```python
from build123d import *

# Parameters (mm, degrees)
SKETCH4_W                          = 6
SKETCH4_H                          = 4.5
BODY_EXTRUDE2_DEPTH                = 6
BODY_SHELL1_T                      = -0.58
BODY_SHELL1_THICKNESS_2_FACE_W     = 3.34
BODY_SHELL1_THICKNESS_2_FACE_H     = 4.84
BODY_SHELL1_THICKNESS_2_DEPTH      = 1.42
EXTRUDE3_REACH                     = 9.075
SKETCH66_W                         = 0.89
SKETCH66_H                         = 1.96
EXTRUDE3_DIRECTION_2_REACH         = 9.075
EXTRUDE2_REACH                     = 9.77
SKETCH65_W                         = 0.5
SKETCH65_H                         = 4
SKETCH65_W_2                       = 1
SKETCH65_H_2                       = 2.5
SKETCH64_W                         = 0.508
SKETCH64_H                         = 0.508
PINS_EXTRUDE_DEPTH                 = 7.045
PINS_CHAMFER_SIZE                  = 0.15
PINS_LPATTERN_COUNT                = 2
PINS_LPATTERN_PITCH                = 2
PINS_CHAMFER_OF_PINS_LPATTERN_SIZE = 0.15


with BuildPart() as part:
    # Sketch4 → Body-Extrude2 (new body)
    with BuildSketch(Plane(origin=(6.86422654, 0, 1.863703399), x_dir=(1, 0, 0), z_dir=(0, 1, 0))):
        with Locations((-6.86422654, 1.863703399)):
            Rectangle(SKETCH4_W, SKETCH4_H)
    extrude(amount=BODY_EXTRUDE2_DEPTH)

    # Body-Shell1
    body_shell1_openings = [part.faces().sort_by_distance(p)[0] for p in [
        (0, 6, 0),
    ]]
    offset(amount=BODY_SHELL1_T, openings=body_shell1_openings, kind=Kind.INTERSECTION)

    # Body-Shell1 thickness 2 face (on inner face of the shell) → Body-Shell1 thickness 2 (add)
    with BuildSketch(Plane(origin=(0, 0.58, 0), x_dir=(0, 0, -1), z_dir=(0, -1, 0))):
        Rectangle(BODY_SHELL1_THICKNESS_2_FACE_W, BODY_SHELL1_THICKNESS_2_FACE_H)
    extrude(amount=-BODY_SHELL1_THICKNESS_2_DEPTH)

    # Extrude3: up to this face of the body (flat: up to its plane)
    extrude3_end = Plane(part.part.faces().sort_by_distance((-3, 3, 0))[0])
    # Sketch66 → Extrude3 (cut, up to the picked face)
    with BuildSketch(Plane(origin=(0, 0, 0), x_dir=(0, 0, -1), z_dir=(1, 0, 0)), mode=Mode.PRIVATE) as extrude3_sk1:
        with Locations((-0.355, 5.02)):
            Rectangle(SKETCH66_W, SKETCH66_H)
    extrude3_tool1 = split(extrude(extrude3_sk1.sketch, amount=-EXTRUDE3_REACH, mode=Mode.PRIVATE), bisect_by=extrude3_end, keep=Keep.BOTH, mode=Mode.PRIVATE)
    add(extrude3_tool1.solids().sort_by(Axis((0, 5.02, 0.355), (-1, 0, 0)))[0], mode=Mode.SUBTRACT)

    # Extrude3 direction 2: up to this face of the body (flat: up to its plane)
    extrude3_direction_2_end = Plane(part.part.faces().sort_by_distance((3, 3, 0))[0])
    # Sketch66 → Extrude3 direction 2 (cut, up to the picked face)
    with BuildSketch(Plane(origin=(0, 0, 0), x_dir=(0, 0, -1), z_dir=(1, 0, 0)), mode=Mode.PRIVATE) as extrude3_direction_2_sk1:
        with Locations((-0.355, 5.02)):
            Rectangle(SKETCH66_W, SKETCH66_H)
    extrude3_direction_2_tool1 = split(extrude(extrude3_direction_2_sk1.sketch, amount=EXTRUDE3_DIRECTION_2_REACH, mode=Mode.PRIVATE), bisect_by=extrude3_direction_2_end, keep=Keep.BOTH, mode=Mode.PRIVATE)
    add(extrude3_direction_2_tool1.solids().sort_by(Axis((0, 5.02, 0.355), (1, 0, 0)))[0], mode=Mode.SUBTRACT)

    # Sketch65 → Extrude2 (cut, up to next)
    with BuildSketch(Plane(origin=(0, 0, 1.67), x_dir=(1, 0, 0), z_dir=(0, 0, -1)), mode=Mode.PRIVATE) as extrude2_sk1:
        with Locations((0, -4)):
            Rectangle(SKETCH65_W, SKETCH65_H)
    extrude2_tool1 = extrude(extrude2_sk1.sketch, amount=-EXTRUDE2_REACH, mode=Mode.PRIVATE) & part.part
    # Sketch65 → Extrude2 (cut, up to next)
    with BuildSketch(Plane(origin=(0, 0, 1.67), x_dir=(1, 0, 0), z_dir=(0, 0, -1)), mode=Mode.PRIVATE) as extrude2_sk2:
        with Locations((-1.92, -3.25)):
            Rectangle(SKETCH65_W_2, SKETCH65_H_2)
    extrude2_tool2 = extrude(extrude2_sk2.sketch, amount=-EXTRUDE2_REACH, mode=Mode.PRIVATE) & part.part
    # Sketch65 → Extrude2 (cut, up to next)
    with BuildSketch(Plane(origin=(0, 0, 1.67), x_dir=(1, 0, 0), z_dir=(0, 0, -1)), mode=Mode.PRIVATE) as extrude2_sk3:
        with Locations((1.92, -3.25)):
            Rectangle(SKETCH65_W_2, SKETCH65_H_2)
    extrude2_tool3 = extrude(extrude2_sk3.sketch, amount=-EXTRUDE2_REACH, mode=Mode.PRIVATE) & part.part
    add(extrude2_tool1.solids().sort_by_distance((0, 4, 1.67))[0], mode=Mode.SUBTRACT)
    add(extrude2_tool2.solids().sort_by_distance((-1.92, 3.25, 1.67))[0], mode=Mode.SUBTRACT)
    add(extrude2_tool3.solids().sort_by_distance((1.92, 3.25, 1.67))[0], mode=Mode.SUBTRACT)

    # Sketch64 → Pins-Extrude (add)
    with BuildSketch(Plane(origin=(0, 5.14, -3.64), x_dir=(1, 0, 0), z_dir=(0, -1, 0))):
        with Locations((1.05, 4.19)):
            Rectangle(SKETCH64_W, SKETCH64_H)
    pins_extrude = extrude(amount=PINS_EXTRUDE_DEPTH)

    # Pins-Chamfer
    pins_chamfer_edges = [part.edges().sort_by_distance(p)[0] for p in [
        (0.796, 5.14, 0.55),
        (1.05, 5.14, 0.296),
        (1.304, 5.14, 0.55),
        (1.05, 5.14, 0.804),
        (1.05, -1.905, 0.804),
        (0.796, -1.905, 0.55),
        (1.05, -1.905, 0.296),
        (1.304, -1.905, 0.55),
    ]]
    chamfer(pins_chamfer_edges, length=PINS_CHAMFER_SIZE)

    # Pins-LPattern: Pins-Extrude ×2
    with Locations(*[(-i * PINS_LPATTERN_PITCH, 0, 0) for i in range(1, PINS_LPATTERN_COUNT)]):
        add(pins_extrude)

    # Pins-Chamfer of Pins-LPattern
    pins_chamfer_of_pins_lpattern_edges = [part.edges().sort_by_distance(p)[0] for p in [
        (-1.204, 5.14, 0.55),
        (-0.95, 5.14, 0.296),
        (-0.696, 5.14, 0.55),
        (-0.95, 5.14, 0.804),
        (-0.95, -1.905, 0.804),
        (-1.204, -1.905, 0.55),
        (-0.95, -1.905, 0.296),
        (-0.696, -1.905, 0.55),
    ]]
    chamfer(pins_chamfer_of_pins_lpattern_edges, length=PINS_CHAMFER_OF_PINS_LPATTERN_SIZE)


solid = part.part
```
Design review of the part built by this model. Coordinates are the model's own, in mm. A direction names the side the tool comes from. Give positions to 0.01 mm unless a question says otherwise; leave off trailing zeros. Order: outer loops, then holes, each group sorted by start corner. A loop starts at its lowest first (then second) coordinate and runs counter-clockwise, first axis right, second up. Notation, with made-up numbers: (-9, -24) -> (39, -24) arc R23 cw to (39, 13) -> close; hole circle Ø2 at (-40, 77). An arc over 180 degrees is marked (long way). Write each question's results on one line, items separated by ' | '. Start each with the question number.
Q1. Add section A-A on x = 2.2. Give the boundary of the cut face in (y, z), and give its area (3 significant figures).
Q2. Machinability: for faces 1 (the flat face through (0, 6, -2)), 2 (the flat face through (-1, 4, 1.67)), which of the approach directions +Z, -Z, +X, -X, +Y, -Y give a long, thin tool a straight path to every point of the face, cutting with its end or side? Answer none if there is none.
Q3. Add section D-D on y = -0.75. Give the boundary of the cut face in (x, z), and give its area (3 significant figures).
Q4. For pin 1 (0.6 mm diameter, centred on x = -2, z = 2, fed in from -Y), flat-tipped, find the tip position at first contact; note if it passes through.
Q5. Wall thickness on L1, parallel to X at y = 4, z = 0.5; L2, parallel to X at y = 5, z = -1.5; L3, parallel to Z at x = -0.9, y = 3: over which ranges is each line inside the solid? List them lowest first. Write a range as from..to.
Q6. Mouldability with a two-part tool opening along Z and no side actions: class faces 3 (the flat face through (0, 3, -2.25)), 4 (the flat face through (0, 0, 0)), 5 (the flat face through (2.42, 3.5, 0.3)), 6 (the flat face through (0, 4, -1.67)) as +Z half, -Z half, draft (parallel to the pull), parting line (faces both ways), or undercut.
Q7. Add section C-C on y = 3. Give the boundary of the cut face in (x, z).
Q8. Add section B-B on y = 5.25. Give the boundary of the cut face in (x, z).
Found:
1) outline: (0, -2.25) -> (6, -2.25) -> (6, -1.67) -> (2, -1.67) -> (2, 2.25) -> (0, 2.25) -> close; (4.5, 1.67) -> (6, 1.67) -> (6, 2.25) -> (4.5, 2.25) -> close | area: 12.2 mm2
2) face 1: +Z, -Z, +X, -X, +Y | face 2: +Y
3) outline: (-1.2, 0.3) -> (-0.7, 0.3) -> (-0.7, 0.8) -> (-1.2, 0.8) -> close; (0.8, 0.3) -> (1.3, 0.3) -> (1.3, 0.8) -> (0.8, 0.8) -> close | area: 0.516 mm2
4) pin 1: stops at y = 0
5) L1: x = -3..-2.42, -1.2..-0.7, 0.8..1.3, 2.42..3 | L2: x = -3..-2.42, 2.42..3 | L3: z = -2.25..-1.67, 0.3..0.8, 1.67..2.25
6) face 3: -Z half | face 4: draft | face 5: undercut | face 6: undercut
7) outline: (-3, -2.25) -> (3, -2.25) -> (3, 2.25) -> (2.42, 2.25) -> (2.42, -1.67) -> (-2.42, -1.67) -> (-2.42, 2.25) -> (-3, 2.25) -> close; (-1.42, 1.67) -> (-0.25, 1.67) -> (-0.25, 2.25) -> (-1.42, 2.25) -> close; (-1.2, 0.3) -> (-0.7, 0.3) -> (-0.7, 0.8) -> (-1.2, 0.8) -> close; (0.25, 1.67) -> (1.42, 1.67) -> (1.42, 2.25) -> (0.25, 2.25) -> close; (0.8, 0.3) -> (1.3, 0.3) -> (1.3, 0.8) -> (0.8, 0.8) -> close
8) outline: (-3, -2.25) -> (3, -2.25) -> (3, -0.09) -> (2.42, -0.09) -> (2.42, -1.67) -> (-2.42, -1.67) -> (-2.42, -0.09) -> (-3, -0.09) -> close; (-3, 0.8) -> (-2.42, 0.8) -> (-2.42, 1.67) -> (-0.25, 1.67) -> (-0.25, 2.25) -> (-3, 2.25) -> close; (0.25, 1.67) -> (2.42, 1.67) -> (2.42, 0.8) -> (3, 0.8) -> (3, 2.25) -> (0.25, 2.25) -> close
